Autodesk Inventor part; units mm, degrees
ref_plane "YZ Plane" through (0, 0, 0) normal (1, 0, 0) x (0, 1, 0)
ref_plane "XZ Plane" through (0, 0, 0) normal (0, 1, 0) x (-1, 0, 0)
ref_plane "XY Plane" through (0, 0, 0) normal (0, 0, 1) x (1, 0, 0)
sketch "Sketch1" plane through (0, 0, 0) normal (0, 1, 0) x (-1, 0, 0)
  line L0 (6.35, 0) -> (501.65, 0)
  line L1 (508, 6.35) -> (508, 349.25)
  line L2 (501.65, 355.6) -> (6.35, 355.6)
  line L3 (0, 349.25) -> (0, 6.35)
  line L4 (374.65, 344.4875) -> (133.35, 344.4875) construction
  line L5 (133.35, 344.4875) -> (133.35, 11.1125) construction
  line L6 (133.35, 11.1125) -> (374.65, 11.1125) construction
  line L7 (374.65, 11.1125) -> (374.65, 344.4875) construction
  line L8 (254, 344.4875) -> (254, 11.1125) construction
  line L9 (374.65, 344.4875) -> (508, 344.4875) construction
  line L10 (374.65, 344.4875) -> (374.65, 355.6) construction
  line L11 (133.35, 11.1125) -> (0, 11.1125) construction
  line L12 (133.35, 11.1125) -> (133.35, 0) construction
  circle A0 centre (374.65, 344.4875) radius 3.175
  circle A1 centre (374.65, 11.1125) radius 3.175
  circle A2 centre (133.35, 11.1125) radius 3.175
  circle A3 centre (133.35, 344.4875) radius 3.175
  circle A4 centre (254, 344.4875) radius 5.5562
  circle A5 centre (254, 11.1125) radius 5.5563
  arc A6 (508, 349.25) -> (501.65, 355.6) centre (501.65, 349.25) ccw
  arc A7 (501.65, 0) -> (508, 6.35) centre (501.65, 6.35) ccw
  arc A8 (0, 6.35) -> (6.35, 0) centre (6.35, 6.35) ccw
  arc A9 (6.35, 355.6) -> (0, 349.25) centre (6.35, 349.25) ccw
  point P0 (0, 0)
  point P1 (508, 355.6)
  point P2 (508, 0)
  point P3 (0, 355.6)
  dimension "d0" = 508
  dimension "d1" = 355.6
  dimension "d2" = 333.375
  dimension "d3" = 241.3
  dimension "d4" = 6.35
  dimension "d5" = 6.35
  dimension "d6" = 6.35
  dimension "d7" = 6.35
  dimension "d8" = 11.1125
  dimension "d9" = 11.1125
  dimension "d10" = 6.35
extrude "Extrusion1" add sketch "Sketch1" along normal blind 1.5875
equation "\"d5\" = d4"
equation "\"d6\" = d4"
equation "\"d7\" = d4"
equation "\"d9\" = d8"
properties part number "14x20 ATNT Sign"
For this review, take the finished solid that the model builds, in its own axes (mm). Coordinates: 2 decimals unless noted, no trailing zeros. Write each loop counter-clockwise with the first axis right and the second up, starting at its lowest first coordinate (ties: lowest second). Pieces come first, ordered by that corner, then holes. Notation, with made-up numbers: (16, 38.25) - (32, 38.25) arc R16 ccw to (32, 47.25) - close; hole circle Ø3 at (-30.75, 28). An arc over 180 degrees is marked (long way). Put each result on its own line as item: value.
1. Mouldability with a two-part tool opening along Z and no side actions: class faces 1 (the cylindrical face through (-248.45, 0.78, 10.87)), 2 (the flat face through (-250, 1.588, 180)) as released by +Z, released by -Z, zero draft, split by the parting line, or undercut.
Values found:
face 1: undercut
face 2: zero draft
2. Wall thickness on probe 1 along Z at (x, y) = (-254, 1.05); probe 2 along Z at (x, y) = (-374.65, 1); probe 3 along X at (y, z) = (1, 15): over which ranges is each line inside the solid? List them lowest first.
Values found:
probe 1: 0 to 5.56, 16.67 to 338.93, 350.04 to 355.6
probe 2: 0 to 7.94, 14.29 to 341.31, 347.66 to 355.6
probe 3: -508 to -257.97, -250.03 to 0
3. Add section A-A, the plane x = -254. Give the boundary of the cut face in (y, z), then the cut area to 3 significant figures.
Values found:
outline: (0, 0) - (1.59, 0) - (1.59, 5.56) - (0, 5.56) - close; (0, 16.67) - (1.59, 16.67) - (1.59, 338.93) - (0, 338.93) - close; (0, 350.04) - (1.59, 350.04) - (1.59, 355.6) - (0, 355.6) - close
area: 529 mm²
4. For pin 1 (10 mm diameter, centred on x = -254, z = 11.11, fed in from +Y), flat-tipped, find the tip position at first contact; note if it passes through.
Values found:
pin 1: through
